Design review of the part shown in the three views and the two pictorial views. Dimensions are in mm from the part's minimum x, y and z. Round coordinates to 2 decimals unless told otherwise and drop trailing zeros. Write each loop counter-clockwise with the first axis right and the second up, starting at its lowest first coordinate (ties: lowest second). Pieces come first, ordered by that corner, then holes. Notation, with made-up numbers: (11, 88.25) -> (54, 88.25) arc R6 cw to (54, 96.25) -> close; hole circle Ø10 at (-5.75, 56.5). An arc over 180 degrees is marked (long way). One line per question, with ' | ' between items. Start each with the question number.
1) Consider section A-A (x = 31). Give the boundary of the cut face in (y, z).
2) Consider section C-C (z = 11). Give the boundary of the cut face in (x, y), then the cut area to 3 significant figures.
3) Consider section D-D (y = 54.5). Give the boundary of the cut face in (x, z), then the cut area to 3 significant figures.
4) Insertion check: pin 1 Ø3 at (y, z) = (25.5, 2.5) entering from -X; pin 2 Ø12 at (x, y) = (13, 44.5) entering from +Z; pin 3 Ø1 at (x, z) = (21.5, 12) entering from -Y. Each pin has a flat end and moves straight along its axis. Give the tip position at first contact, or say it passes through.
5) Consider section B-B (y = 30). Give the boundary of the cut face in (x, z), then the cut area to 3 significant figures.
6) For probe 1 along Z at (x, y) = (61.5, 5), list the stretches that pass through material, from the lowest coordinate up.
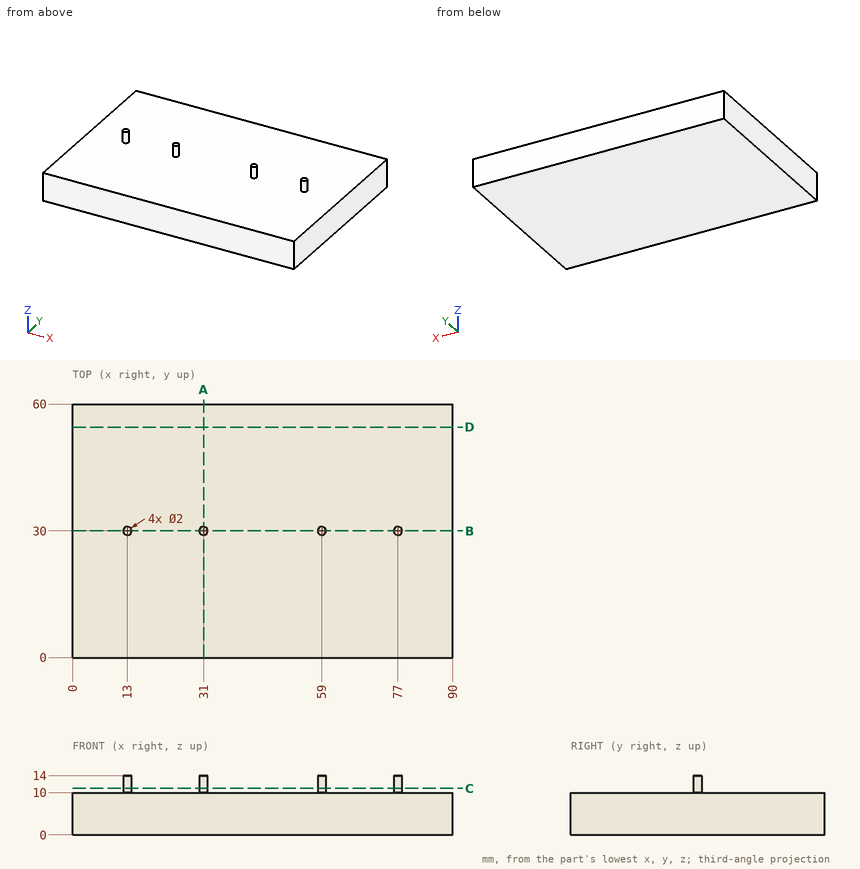
From the geometry:
1) outline: (0, 0) -> (60, 0) -> (60, 10) -> (31, 10) -> (31, 14) -> (29, 14) -> (29, 10) -> (0, 10) -> close
2) outline: circle Ø2 at (13, 30); circle Ø2 at (31, 30); circle Ø2 at (59, 30); circle Ø2 at (77, 30) | area: 12.6 mm2
3) outline: (0, 0) -> (90, 0) -> (90, 10) -> (0, 10) -> close | area: 900 mm2
4) pin 1: stops at x = 0 | pin 2: stops at z = 10 | pin 3: passes through
5) outline: (0, 0) -> (90, 0) -> (90, 10) -> (78, 10) -> (78, 14) -> (76, 14) -> (76, 10) -> (60, 10) -> (60, 14) -> (58, 14) -> (58, 10) -> (32, 10) -> (32, 14) -> (30, 14) -> (30, 10) -> (14, 10) -> (14, 14) -> (12, 14) -> (12, 10) -> (0, 10) -> close | area: 932 mm2
6) probe 1: z = 0 to 10
